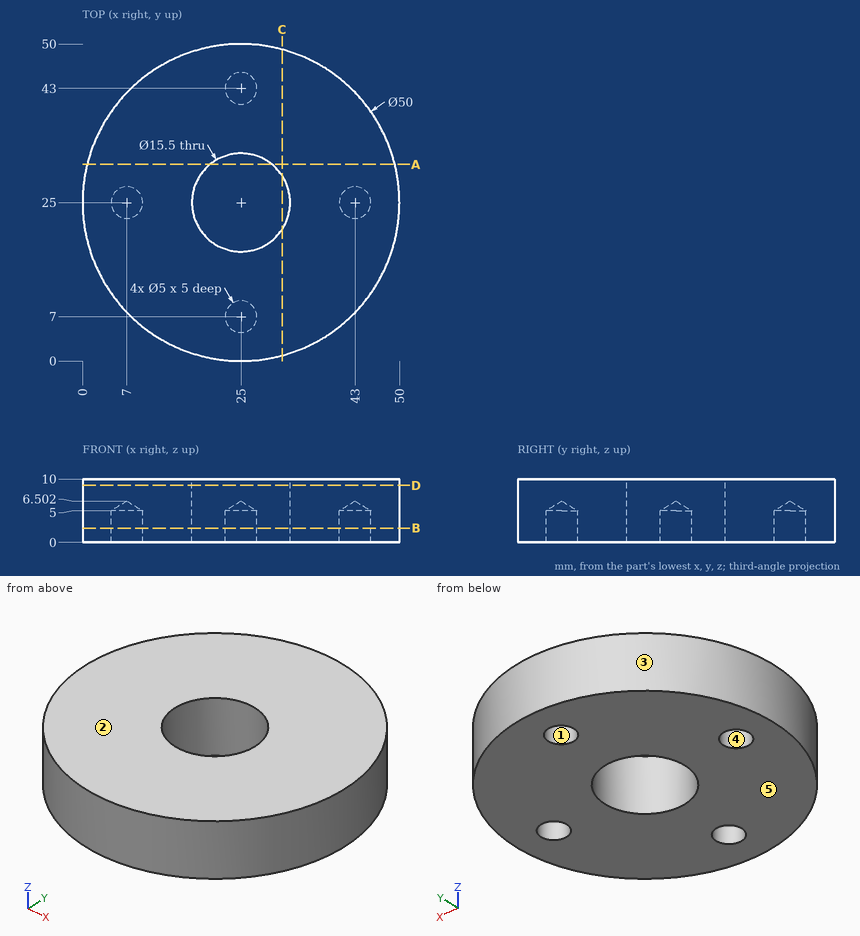
The drawing under review shows one solid part. Ordinate dimensions are in mm from its lowest x, y, z. A direction names the side the tool comes from. Round coordinates to 2 decimals unless told otherwise and drop trailing zeros. Loops run counter-clockwise (first coordinate to the right, second up) from the corner with the lowest first, then second, coordinate; pieces in that order, holes last. Notation, with made-up numbers: (8.25, 36.5) -> (64.25, 36.5) arc R36 ccw to (64.25, 70.5) -> close; hole circle Ø7 at (-7, 13.5). An arc over 180 degrees is marked (long way). Answer in a Markdown table with one row per item.
1) Wall thickness on line 1 along Y through (x, z) = (25, 1.7); line 2 along Y through (x, z) = (25, 6.75); line 3 along Y through (x, z) = (43, 3.25): over which ranges is each line inside the solid? List them lowest first.
Taken from the geometry:
| item | result |
|---|---|
| line 1 | y = 0 to 4.5, 9.5 to 17.25, 32.75 to 40.5, 45.5 to 50 |
| line 2 | y = 0 to 17.25, 32.75 to 50 |
| line 3 | y = 7.65 to 22.5, 27.5 to 42.35 |
2) Consider section A-A, the plane y = 31. Write out the cut boundary in (x, z), plus the area to 3 significant figures.
Taken from the geometry:
| item | result |
|---|---|
| outline | (0.73, 0) -> (20.09, 0) -> (20.09, 10) -> (0.73, 10) -> close; (29.91, 0) -> (49.27, 0) -> (49.27, 10) -> (29.91, 10) -> close |
| area | 387 mm² |
3) Consider section D-D, the plane z = 9. Write out the cut boundary in (x, y), plus the area to 3 significant figures.
Taken from the geometry:
| item | result |
|---|---|
| outline | circle Ø50 at (25, 25); hole circle Ø15.5 at (25, 25) |
| area | 1,770 mm² |
4) Tool access review of the marked faces 1 and 2: name each direction out of +Z, -Z, +X, -X, +Y, -Y from which nothing blocks a thin tool from reaching the whole face with its end or side.
Taken from the geometry:
| item | result |
|---|---|
| face 1 | -Z |
| face 2 | +Z, +X, -X, +Y, -Y |
5) Draft analysis for pull direction X (two halves, no side actions). For the marked faces 3, 4 and 5, state which applies: pulls with the +X half, pulls with the -X half, needs draft (parallel to the pull), parting line crosses it, or undercut.
Taken from the geometry:
| item | result |
|---|---|
| face 3 | parting line crosses it |
| face 4 | undercut |
| face 5 | needs draft |
6) Consider section C-C, the plane x = 31.5. Write out the cut boundary in (y, z), plus the area to 3 significant figures.
Taken from the geometry:
| item | result |
|---|---|
| outline | (0.86, 0) -> (20.78, 0) -> (20.78, 10) -> (0.86, 10) -> close; (29.22, 0) -> (49.14, 0) -> (49.14, 10) -> (29.22, 10) -> close |
| area | 398 mm² |
7) For pin 1 Ø5 at (x, z) = (13, 8) entering from +Y (1 decimal); pin 2 Ø4 at (y, z) = (21, 7) entering from +X; pin 3 Ø2 at (x, z) = (44.5, 2) entering from +Y (1 decimal), all flat-tipped, find the tip position at first contact; note any pin that passes through.
Taken from the geometry:
| item | result |
|---|---|
| pin 1 | stops at y = 48.1 |
| pin 2 | stops at x = 49.92 |
| pin 3 | stops at y = 41.8 |
8) Consider section B-B, the plane z = 2.25. Write out the cut boundary in (x, y), plus the area to 3 significant figures.
Taken from the geometry:
| item | result |
|---|---|
| outline | circle Ø50 at (25, 25); hole circle Ø5 at (7, 25); hole circle Ø15.5 at (25, 25); hole circle Ø5 at (25, 7); hole circle Ø5 at (25, 43); hole circle Ø5 at (43, 25) |
| area | 1,700 mm² |
